Input: part model. Units: mm. Frame: model coordinates. Face numbers are marked on the shaded views. A direction names the side the tool comes from. Coordinates: 2 decimals unless noted, no trailing zeros. Loops run counter-clockwise (first coordinate to the right, second up) from the corner with the lowest first, then second, coordinate; pieces in that order, holes last. Notation, with made-up numbers: (-18.75, 10.5) - (25.25, 10.5) arc R17 cw to (25.25, 25.5) - close; hole circle Ø5 at (-10, 29.5). An arc over 180 degrees is marked (long way). Use one line per item in the form item = value.
from build123d import *

# Parameters (mm, degrees)
F0_W     = 5
F0_H     = 5
F1_DEPTH = 5
F2_R     = 1.45
F3_DEPTH = 5.001
F4_W     = 5
F4_H     = 5
F4_W_2   = 2.2
F4_H_2   = 3.7
F5_DEPTH = 3
F6_DEPTH = 1


with BuildPart() as f1:
    # F0 (on Top) → F1 (new body)
    with BuildSketch(Plane.XY):
        Rectangle(F0_W, F0_H)
    extrude(amount=F1_DEPTH)

    # F2 (on face) → F3 (cut, through all)
    with BuildSketch(Plane.XY.offset(5)):
        Circle(F2_R)
    extrude(amount=-F3_DEPTH, mode=Mode.SUBTRACT)

    # F4 (on face) → F5 (join)
    with BuildSketch(Plane.XY.offset(5)):
        Rectangle(F4_W, F4_H)
        Rectangle(F4_W_2, F4_H_2, mode=Mode.SUBTRACT)
    extrude(amount=F5_DEPTH)

    # F4 (on face) → F6 (join)
    with BuildSketch(Plane.XY.offset(5)):
        Rectangle(F4_W, F4_H)
        with BuildLine():
            Line((1.1, -0.9447221814), (1.1, -1.85))
            Line((1.1, -1.85), (-1.1, -1.85))
            Line((-1.1, -1.85), (-1.1, -0.9447221814))
            ThreePointArc((-1.1, -0.9447221814), (-1.45, 0), (-1.1, 0.9447221814))
            Line((-1.1, 0.9447221814), (-1.1, 1.85))
            Line((-1.1, 1.85), (1.1, 1.85))
            Line((1.1, 1.85), (1.1, 0.9447221814))
            ThreePointArc((1.1, 0.9447221814), (1.3596874641, 0.503736042), (1.45, 0))
            ThreePointArc((1.45, 0), (1.3596874641, -0.503736042), (1.1, -0.9447221814))
        make_face(mode=Mode.SUBTRACT)
        with BuildLine():
            ThreePointArc((-1.1, 0.9447221814), (0, 1.45), (1.1, 0.9447221814))
            Line((1.1, 0.9447221814), (1.1, 1.85))
            Line((1.1, 1.85), (-1.1, 1.85))
            Line((-1.1, 1.85), (-1.1, 0.9447221814))
        make_face()
        with BuildLine():
            ThreePointArc((-1.1, 0.9447221814), (-1.45, 0), (-1.1, -0.9447221814))
            Line((-1.1, -0.9447221814), (-1.1, 0.9447221814))
        make_face()
        with BuildLine():
            ThreePointArc((-1.1, -0.9447221814), (0, -1.45), (1.1, -0.9447221814))
            Line((1.1, -0.9447221814), (1.1, 0.9447221814))
            ThreePointArc((1.1, 0.9447221814), (0, 1.45), (-1.1, 0.9447221814))
            Line((-1.1, 0.9447221814), (-1.1, -0.9447221814))
        make_face()
        with BuildLine():
            Line((1.1, 0.9447221814), (1.1, -0.9447221814))
            ThreePointArc((1.1, -0.9447221814), (1.3596874641, -0.503736042), (1.45, 0))
            ThreePointArc((1.45, 0), (1.3596874641, 0.503736042), (1.1, 0.9447221814))
        make_face()
        with BuildLine():
            Line((-1.1, -1.85), (1.1, -1.85))
            Line((1.1, -1.85), (1.1, -0.9447221814))
            ThreePointArc((1.1, -0.9447221814), (0, -1.45), (-1.1, -0.9447221814))
            Line((-1.1, -0.9447221814), (-1.1, -1.85))
        make_face()
    extrude(amount=-F6_DEPTH)


solid = f1.part
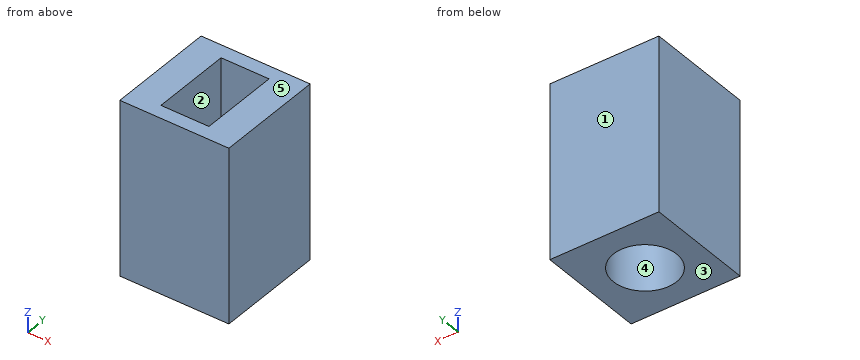
Q1. Set-up query: the marked faces 1 and 2. Return all of +Z, -Z, +X, -X, +Y, -Y with unobstructed straight access to the full face (end or side cutting, diameter ignored); none if empty.
Check values:
face_1 = +Z, -Z, +X, -X, +Y
face_2 = +Z
Q2. Cut plane C-C, the plane x = 0. Return loops of the section in (y, z), then the cut area to 3 significant figures.
Check values:
outline = (-2.5, 0) - (-1.45, 0) - (-1.45, 4) - (1.45, 4) - (1.45, 0) - (2.5, 0) - (2.5, 8) - (1.85, 8) - (1.85, 5) - (-1.85, 5) - (-1.85, 8) - (-2.5, 8) - close
area = 17.3 mm²
Q3. Cut plane B-B, the plane y = 0. Return loops of the section in (x, z), then the cut area to 3 significant figures.
Check values:
outline = (-2.5, 0) - (-1.45, 0) - (-1.45, 4) - (1.45, 4) - (1.45, 0) - (2.5, 0) - (2.5, 8) - (1.1, 8) - (1.1, 5) - (-1.1, 5) - (-1.1, 8) - (-2.5, 8) - close
area = 21.8 mm²
Q4. Cut plane A-A, the plane z = 7.25. Return loops of the section in (x, y).
Check values:
outline = (-2.5, -2.5) - (2.5, -2.5) - (2.5, 2.5) - (-2.5, 2.5) - close; hole (-1.1, -1.85) - (1.1, -1.85) - (1.1, 1.85) - (-1.1, 1.85) - close
Q5. First-contact query: P1, Ø1.8, axis at x = 0, y = 0.5, coming from the +Z side. Flat tip, straight axial feed; report the tip coordinate or a pass-through.
Check values:
P1 = 5
Q6. Ray query, line 1 along X through (y, z) = (0.5, 5.25); line 2 along Y through (x, z) = (0, 1.85); line 3 along Y through (x, z) = (0.6, 7). Return the intervals inside material, ascending. Write a range as [from, to].
Check values:
line_1 = [-2.5, -1.1], [1.1, 2.5]
line_2 = [-2.5, -1.45], [1.45, 2.5]
line_3 = [-2.5, -1.85], [1.85, 2.5]
Q7. Pull-direction query (Z, two-part tool) for the marked faces 3, 4 and 5; classes: pulls with the +Z half, pulls with the -Z half, needs draft (parallel to the pull), parting line crosses it, or undercut.
Check values:
face_3 = pulls with the -Z half
face_4 = needs draft
face_5 = pulls with the +Z half
Q8. Cut plane D-D, the plane z = 3.25. Return loops of the section in (x, y), then the cut area to 3 significant figures.
Check values:
outline = (-2.5, -2.5) - (2.5, -2.5) - (2.5, 2.5) - (-2.5, 2.5) - close; hole circle Ø2.9 at (0, 0)
area = 18.4 mm²
